Model file for the job. Use its own axes, mm. Face numbers are marked on the shaded views. A direction names the side the tool comes from. Round coordinates to 2 decimals unless told otherwise and drop trailing zeros. Loops run counter-clockwise (first coordinate to the right, second up) from the corner with the lowest first, then second, coordinate; pieces in that order, holes last. Notation, with made-up numbers: (-18.5, 30.25) - (17.5, 30.25) arc R24 ccw to (17.5, 64.25) - close; hole circle Ø4 at (29, 53.5). An arc over 180 degrees is marked (long way). Use one line per item in the form item = value.
from build123d import *

# Parameters (mm, degrees)
SKETCH1_W                      = 38.1
SKETCH1_H                      = 48.26
SKETCH1_W_2                    = 31.75
SKETCH1_H_2                    = 41.91
BOSS_EXTRUDE1_DEPTH            = 152.4
SKETCH2_R                      = 1.89865
CUT_EXTRUDE1_DEPTH             = 35.925
CUT_EXTRUDE1_DEPTH_BACK        = 4.175
CUT_EXTRUDE3_DEPTH             = 3.175
CUT_EXTRUDE4_DEPTH             = 3.175
CUT_EXTRUDE5_REACH             = 36.925
SKETCH6_R                      = 9.525
SKETCH6_R_2                    = 2.5527
CUT_EXTRUDE6_DEPTH             = 3.175
F_6_32_TAPPED_HOLE2_D          = 2.7051
F_6_32_TAPPED_HOLE2_DEPTH      = 3.175
CUT_EXTRUDE7_REACH             = 40.1
CUT_EXTRUDE7_DIRECTION_2_DEPTH = 1
FILLET1_R                      = 3.175
FILLET2_R                      = 3.175
BOSS_EXTRUDE2_DEPTH            = 3.175
CUT_EXTRUDE8_REACH             = 40.1
FILLET3_R                      = 3.175
FILLET4_R                      = 3.175
FILLET5_R                      = 6.35
FILLET6_R                      = 6.35
BOSS_EXTRUDE3_DEPTH            = 3.175
CUT_EXTRUDE9_REACH             = 40.1
BOSS_EXTRUDE4_DEPTH            = 3.175
FILLET7_R                      = 3.175
FILLET8_R                      = 3.175
FILLET9_R                      = 3.175
FILLET10_R                     = 3.175
FILLET11_R                     = 6.35
FILLET12_R                     = 6.35


with BuildPart() as part:
    # Sketch1 → Boss-Extrude1 (new body)
    with BuildSketch(Plane(origin=(0, 0, 0), x_dir=(1, 0, 0), z_dir=(0, 1, 0))):
        Rectangle(SKETCH1_W, SKETCH1_H)
        Rectangle(SKETCH1_W_2, SKETCH1_H_2, mode=Mode.SUBTRACT)
    extrude(amount=BOSS_EXTRUDE1_DEPTH)

    # Sketch2 → Cut-Extrude1 (cut, two sides)
    with BuildSketch(Plane(origin=(-15.875, 0, 0), x_dir=(0, 0, -1), z_dir=(1, 0, 0))) as cut_extrude1_sk:
        with Locations((-16.645384182, 6.21538)):
            Circle(SKETCH2_R)
        with Locations((10.30030417, 6.18241423)):
            Circle(SKETCH2_R)
    extrude(amount=CUT_EXTRUDE1_DEPTH, mode=Mode.SUBTRACT)
    extrude(cut_extrude1_sk.sketch, amount=-CUT_EXTRUDE1_DEPTH_BACK, mode=Mode.SUBTRACT)

    # Sketch4 → Cut-Extrude3 (cut)
    with BuildSketch(Plane.ZY.offset(19.05)):
        with BuildLine():
            Line((16.1925, 10.16), (-16.1925, 10.16))
            ThreePointArc((-16.1925, 10.16), (-18.43756403, 11.08993597), (-19.3675, 13.335))
            Line((-19.3675, 13.335), (-19.3675, 64.135))
            ThreePointArc((-19.3675, 64.135), (-18.43756403, 66.38006403), (-16.1925, 67.31))
            Line((-16.1925, 67.31), (16.1925, 67.31))
            ThreePointArc((16.1925, 67.31), (18.43756403, 66.38006403), (19.3675, 64.135))
            Line((19.3675, 64.135), (19.3675, 13.335))
            ThreePointArc((19.3675, 13.335), (18.43756403, 11.08993597), (16.1925, 10.16))
        make_face()
    extrude(amount=-CUT_EXTRUDE3_DEPTH, mode=Mode.SUBTRACT)

    # Sketch5 → Cut-Extrude4 (cut)
    with BuildSketch(Plane(origin=(19.05, 0, 0), x_dir=(0, 0, -1), z_dir=(1, 0, 0))):
        with BuildLine():
            Line((16.1925, 67.31), (-16.1925, 67.31))
            ThreePointArc((-16.1925, 67.31), (-18.43756403, 66.38006403), (-19.3675, 64.135))
            Line((-19.3675, 64.135), (-19.3675, 45.085))
            ThreePointArc((-19.3675, 45.085), (-18.43756403, 42.83993597), (-16.1925, 41.91))
            Line((-16.1925, 41.91), (16.1925, 41.91))
            ThreePointArc((16.1925, 41.91), (18.43756403, 42.83993597), (19.3675, 45.085))
            Line((19.3675, 45.085), (19.3675, 64.135))
            ThreePointArc((19.3675, 64.135), (18.43756403, 66.38006403), (16.1925, 67.31))
        make_face()
    extrude(amount=-CUT_EXTRUDE4_DEPTH, mode=Mode.SUBTRACT)

    # Sketch6 → Cut-Extrude5 (cut, up to next)
    with BuildSketch(Plane(origin=(-15.875, 0, 0), x_dir=(0, 0, -1), z_dir=(1, 0, 0)), mode=Mode.PRIVATE) as cut_extrude5_sk1:
        with Locations((0, 101.6)):
            Circle(SKETCH6_R)
    cut_extrude5_tool1 = extrude(cut_extrude5_sk1.sketch, amount=CUT_EXTRUDE5_REACH, mode=Mode.PRIVATE) & part.part
    add(cut_extrude5_tool1.solids().sort_by_distance((-15.875, 101.6, 0))[0], mode=Mode.SUBTRACT)
    # Sketch6 → Cut-Extrude5 (cut, up to next)
    with BuildSketch(Plane(origin=(-15.875, 0, 0), x_dir=(0, 0, -1), z_dir=(1, 0, 0)), mode=Mode.PRIVATE) as cut_extrude5_sk2:
        with Locations((0, 87.63)):
            Circle(SKETCH6_R_2)
    cut_extrude5_tool2 = extrude(cut_extrude5_sk2.sketch, amount=CUT_EXTRUDE5_REACH, mode=Mode.PRIVATE) & part.part
    add(cut_extrude5_tool2.solids().sort_by_distance((-15.875, 87.63, 0))[0], mode=Mode.SUBTRACT)
    # Sketch6 → Cut-Extrude5 (cut, up to next)
    with BuildSketch(Plane(origin=(-15.875, 0, 0), x_dir=(0, 0, -1), z_dir=(1, 0, 0)), mode=Mode.PRIVATE) as cut_extrude5_sk3:
        with Locations((-9.878281733, 91.721718267)):
            Circle(SKETCH6_R_2)
    cut_extrude5_tool3 = extrude(cut_extrude5_sk3.sketch, amount=CUT_EXTRUDE5_REACH, mode=Mode.PRIVATE) & part.part
    add(cut_extrude5_tool3.solids().sort_by_distance((-15.875, 91.721718, 9.878282))[0], mode=Mode.SUBTRACT)
    # Sketch6 → Cut-Extrude5 (cut, up to next)
    with BuildSketch(Plane(origin=(-15.875, 0, 0), x_dir=(0, 0, -1), z_dir=(1, 0, 0)), mode=Mode.PRIVATE) as cut_extrude5_sk4:
        with Locations((-13.97, 101.6)):
            Circle(SKETCH6_R_2)
    cut_extrude5_tool4 = extrude(cut_extrude5_sk4.sketch, amount=CUT_EXTRUDE5_REACH, mode=Mode.PRIVATE) & part.part
    add(cut_extrude5_tool4.solids().sort_by_distance((-15.875, 101.6, 13.97))[0], mode=Mode.SUBTRACT)
    # Sketch6 → Cut-Extrude5 (cut, up to next)
    with BuildSketch(Plane(origin=(-15.875, 0, 0), x_dir=(0, 0, -1), z_dir=(1, 0, 0)), mode=Mode.PRIVATE) as cut_extrude5_sk5:
        with Locations((-9.878281733, 111.478281733)):
            Circle(SKETCH6_R_2)
    cut_extrude5_tool5 = extrude(cut_extrude5_sk5.sketch, amount=CUT_EXTRUDE5_REACH, mode=Mode.PRIVATE) & part.part
    add(cut_extrude5_tool5.solids().sort_by_distance((-15.875, 111.478282, 9.878282))[0], mode=Mode.SUBTRACT)
    # Sketch6 → Cut-Extrude5 (cut, up to next)
    with BuildSketch(Plane(origin=(-15.875, 0, 0), x_dir=(0, 0, -1), z_dir=(1, 0, 0)), mode=Mode.PRIVATE) as cut_extrude5_sk6:
        with Locations((0, 115.57)):
            Circle(SKETCH6_R_2)
    cut_extrude5_tool6 = extrude(cut_extrude5_sk6.sketch, amount=CUT_EXTRUDE5_REACH, mode=Mode.PRIVATE) & part.part
    add(cut_extrude5_tool6.solids().sort_by_distance((-15.875, 115.57, 0))[0], mode=Mode.SUBTRACT)
    # Sketch6 → Cut-Extrude5 (cut, up to next)
    with BuildSketch(Plane(origin=(-15.875, 0, 0), x_dir=(0, 0, -1), z_dir=(1, 0, 0)), mode=Mode.PRIVATE) as cut_extrude5_sk7:
        with Locations((9.878281733, 111.478281733)):
            Circle(SKETCH6_R_2)
    cut_extrude5_tool7 = extrude(cut_extrude5_sk7.sketch, amount=CUT_EXTRUDE5_REACH, mode=Mode.PRIVATE) & part.part
    add(cut_extrude5_tool7.solids().sort_by_distance((-15.875, 111.478282, -9.878282))[0], mode=Mode.SUBTRACT)
    # Sketch6 → Cut-Extrude5 (cut, up to next)
    with BuildSketch(Plane(origin=(-15.875, 0, 0), x_dir=(0, 0, -1), z_dir=(1, 0, 0)), mode=Mode.PRIVATE) as cut_extrude5_sk8:
        with Locations((13.97, 101.6)):
            Circle(SKETCH6_R_2)
    cut_extrude5_tool8 = extrude(cut_extrude5_sk8.sketch, amount=CUT_EXTRUDE5_REACH, mode=Mode.PRIVATE) & part.part
    add(cut_extrude5_tool8.solids().sort_by_distance((-15.875, 101.6, -13.97))[0], mode=Mode.SUBTRACT)
    # Sketch6 → Cut-Extrude5 (cut, up to next)
    with BuildSketch(Plane(origin=(-15.875, 0, 0), x_dir=(0, 0, -1), z_dir=(1, 0, 0)), mode=Mode.PRIVATE) as cut_extrude5_sk9:
        with Locations((9.878281733, 91.721718267)):
            Circle(SKETCH6_R_2)
    cut_extrude5_tool9 = extrude(cut_extrude5_sk9.sketch, amount=CUT_EXTRUDE5_REACH, mode=Mode.PRIVATE) & part.part
    add(cut_extrude5_tool9.solids().sort_by_distance((-15.875, 91.721718, -9.878282))[0], mode=Mode.SUBTRACT)

    # Sketch7 → Cut-Extrude6 (cut)
    with BuildSketch(Plane.ZY.offset(19.05)):
        with BuildLine():
            Line((-13.0175, 77.47), (13.0175, 77.47))
            ThreePointArc((13.0175, 77.47), (17.507628061, 79.329871939), (19.3675, 83.82))
            Line((19.3675, 83.82), (19.3675, 121.92))
            ThreePointArc((19.3675, 121.92), (17.507628061, 126.410128061), (13.0175, 128.27))
            Line((13.0175, 128.27), (-13.0175, 128.27))
            ThreePointArc((-13.0175, 128.27), (-17.507628061, 126.410128061), (-19.3675, 121.92))
            Line((-19.3675, 121.92), (-19.3675, 83.82))
            ThreePointArc((-19.3675, 83.82), (-17.507628061, 79.329871939), (-13.0175, 77.47))
        make_face()
    extrude(amount=-CUT_EXTRUDE6_DEPTH, mode=Mode.SUBTRACT)

    # #6-32 Tapped Hole2
    with Locations(Plane(origin=(5.579615818, 136.6393, -24.13), x_dir=(-1, 0, 0), z_dir=(0, 0, -1))):
        with Locations((0, 0), (11.159231636, 0)):
            Hole(F_6_32_TAPPED_HOLE2_D / 2, depth=F_6_32_TAPPED_HOLE2_DEPTH)

    # Sketch13 → Cut-Extrude7 (cut, up to next)
    with BuildSketch(Plane(origin=(19.05, 0, 0), x_dir=(0, 0, -1), z_dir=(1, 0, 0)), mode=Mode.PRIVATE) as cut_extrude7_sk1:
        Polygon((0, 78.486), (19.3675, 78.486), (19.3675, 64.135), (-19.3675, 64.135), (-19.3675, 78.486), align=None)
    cut_extrude7_tool1 = extrude(cut_extrude7_sk1.sketch, amount=-CUT_EXTRUDE7_REACH, mode=Mode.PRIVATE) & part.part
    add(cut_extrude7_tool1.solids().sort_by_distance((19.05, 71.3105, 0))[0], mode=Mode.SUBTRACT)

    # Sketch13 → Cut-Extrude7 direction 2 (cut)
    with BuildSketch(Plane(origin=(19.05, 0, 0), x_dir=(0, 0, -1), z_dir=(1, 0, 0))):
        Polygon((0, 78.486), (19.3675, 78.486), (19.3675, 64.135), (-19.3675, 64.135), (-19.3675, 78.486), align=None)
    extrude(amount=CUT_EXTRUDE7_DIRECTION_2_DEPTH, mode=Mode.SUBTRACT)

    # Fillet1
    fillet1_edges = [part.edges().sort_by_distance(p)[0] for p in [
        (17.4625, 78.486, -19.3675),
    ]]
    fillet(fillet1_edges, radius=FILLET1_R)

    # Fillet2
    fillet2_edges = [part.edges().sort_by_distance(p)[0] for p in [
        (17.4625, 78.486, 19.3675),
    ]]
    fillet(fillet2_edges, radius=FILLET2_R)

    # Sketch15 → Boss-Extrude2 (add)
    with BuildSketch(Plane.ZY.offset(19.05)):
        Polygon((0, 78.486), (-19.3675, 78.486), (-19.3675, 88.646), (0, 88.646), (19.3675, 88.646), (19.3675, 78.486), align=None)
    extrude(amount=-BOSS_EXTRUDE2_DEPTH)

    # Sketch16 → Cut-Extrude8 (cut, up to next)
    with BuildSketch(Plane.ZY.offset(19.05), mode=Mode.PRIVATE) as cut_extrude8_sk1:
        Polygon((0, 78.486), (19.3675, 78.486), (19.3675, 64.135), (-19.3675, 64.135), (-19.3675, 78.486), align=None)
    cut_extrude8_tool1 = extrude(cut_extrude8_sk1.sketch, amount=-CUT_EXTRUDE8_REACH, mode=Mode.PRIVATE) & part.part
    add(cut_extrude8_tool1.solids().sort_by_distance((-19.05, 71.3105, 0))[0], mode=Mode.SUBTRACT)

    # Fillet3
    fillet3_edges = [part.edges().sort_by_distance(p)[0] for p in [
        (-17.4625, 78.486, 19.3675),
    ]]
    fillet(fillet3_edges, radius=FILLET3_R)

    # Fillet4
    fillet4_edges = [part.edges().sort_by_distance(p)[0] for p in [
        (-17.4625, 78.486, -19.3675),
    ]]
    fillet(fillet4_edges, radius=FILLET4_R)

    # Fillet5
    fillet5_edges = [part.edges().sort_by_distance(p)[0] for p in [
        (-17.4625, 88.646, -19.3675),
    ]]
    fillet(fillet5_edges, radius=FILLET5_R)

    # Fillet6
    fillet6_edges = [part.edges().sort_by_distance(p)[0] for p in [
        (-17.4625, 88.646, 19.3675),
    ]]
    fillet(fillet6_edges, radius=FILLET6_R)

    # Sketch17 → Boss-Extrude3 (add)
    with BuildSketch(Plane.ZY.offset(19.05)):
        Polygon((0, 74.168), (19.3675, 74.168), (19.3675, 84.35471455), (-20.6375, 84.35471455), (-19.3675, 74.168), align=None)
    extrude(amount=-BOSS_EXTRUDE3_DEPTH)

    # Sketch18 → Cut-Extrude9 (cut, up to next)
    with BuildSketch(Plane.ZY.offset(19.05), mode=Mode.PRIVATE) as cut_extrude9_sk1:
        Polygon((0, 84.328), (-19.3675, 84.328), (-19.3675, 94.996), (19.3675, 94.996), (19.3675, 84.328), align=None)
    cut_extrude9_tool1 = extrude(cut_extrude9_sk1.sketch, amount=-CUT_EXTRUDE9_REACH, mode=Mode.PRIVATE) & part.part
    add(cut_extrude9_tool1.solids().sort_by_distance((-19.05, 89.662, 0))[0], mode=Mode.SUBTRACT)

    # Sketch19 → Boss-Extrude4 (add)
    with BuildSketch(Plane(origin=(19.05, 0, 0), x_dir=(0, 0, -1), z_dir=(1, 0, 0))):
        Polygon((0, 74.168), (19.3675, 74.168), (19.3675, 78.486), (-19.3675, 78.486), (-19.3675, 74.168), align=None)
    extrude(amount=-BOSS_EXTRUDE4_DEPTH)

    # Fillet7
    fillet7_edges = [part.edges().sort_by_distance(p)[0] for p in [
        (17.4625, 74.168, -19.3675),
    ]]
    fillet(fillet7_edges, radius=FILLET7_R)

    # Fillet8
    fillet8_edges = [part.edges().sort_by_distance(p)[0] for p in [
        (17.4625, 74.168, 19.3675),
    ]]
    fillet(fillet8_edges, radius=FILLET8_R)

    # Fillet9
    fillet9_edges = [part.edges().sort_by_distance(p)[0] for p in [
        (-17.4625, 74.168, 19.3675),
    ]]
    fillet(fillet9_edges, radius=FILLET9_R)

    # Fillet10
    fillet10_edges = [part.edges().sort_by_distance(p)[0] for p in [
        (-17.4625, 74.168, -19.3675),
    ]]
    fillet(fillet10_edges, radius=FILLET10_R)

    # Fillet11
    fillet11_edges = [part.edges().sort_by_distance(p)[0] for p in [
        (-17.4625, 84.328, -19.3675),
    ]]
    fillet(fillet11_edges, radius=FILLET11_R)

    # Fillet12
    fillet12_edges = [part.edges().sort_by_distance(p)[0] for p in [
        (-17.4625, 84.328, 19.3675),
    ]]
    fillet(fillet12_edges, radius=FILLET12_R)


solid = part.part
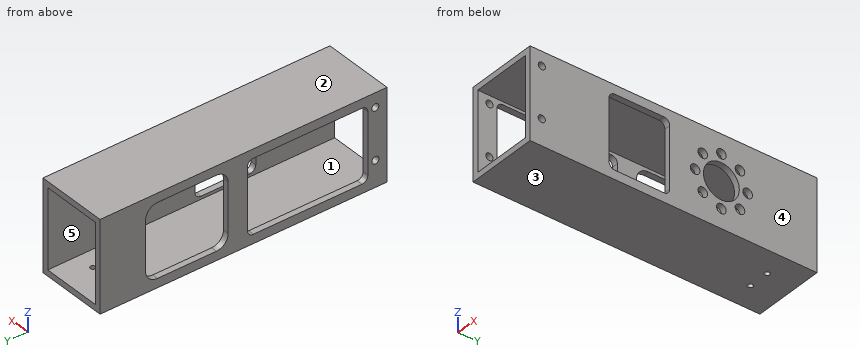
1. Flat gauge pins, fed straight in: pin 1 (3 mm diameter, centred on x = -5.58, y = 136.64, fed in from -Z); pin 2 (2 mm diameter, centred on y = 28.5, z = -8.5, fed in from -X) (3 decimals). Where does each tip first touch, or does it go through?
Geometry check:
pin_1 = -24.13
pin_2 = 15.875
2. Tool access for the marked faces 4 and 5: list every direction of +Z, -Z, +X, -X, +Y, -Y with a clear straight run to the whole face (end or side of a thin tool).
Geometry check:
face_4 = +Z, -Z, +X, +Y, -Y
face_5 = +Y, -Y
3. Cut at B-B, the plane z = 0. Give the number of separate pieces and of enclosed holes in the cut face, plus the area to 3 significant figures.
Geometry check:
separate_pieces = 8
enclosed_holes = 0
area = 430 mm^2
4. Cut at D-D, the plane y = 78. Give the cut face in (x, z) (3 decimals), plus the area to 3 significant figures.
Geometry check:
outline = (-19.05, -24.13) - (19.05, -24.13) - (19.05, 24.13) - (-19.05, 24.13) - close; hole (-15.875, -20.955) - (15.875, -20.955) - (15.875, 20.955) - (-15.875, 20.955) - close
area = 508 mm^2
5. Cut at A-A, the plane x = 1.5. Give the cut face in (y, z) (3 decimals), plus the area to 3 significant figures.
Geometry check:
outline = (0, -24.13) - (152.4, -24.13) - (152.4, -20.955) - (0, -20.955) - close; (0, 20.955) - (152.4, 20.955) - (152.4, 24.13) - (0, 24.13) - close
area = 968 mm^2
6. Wall check: probe 1 along Y at (x, z) = (16.85, 0) (3 decimals); probe 2 along Z at (x, y) = (16.7, 101.6) (3 decimals); probe 3 along X at (y, z) = (6.5, 2) (3 decimals). Give the ranges that are in metal, low to high.
Geometry check:
probe_1 = 0 to 41.91, 74.168 to 85.077, 90.183 to 92.075, 111.125 to 113.017, 118.123 to 152.4
probe_2 = -24.13 to -16.523, -11.417 to -9.525, 9.525 to 11.417, 16.523 to 24.13
probe_3 = -19.05 to -15.875, 15.875 to 19.05
7. Pull direction Z, two halves, no side cores. Call the marked faces 1, 2 and 3: +Z half, -Z half, draft (parallel to the pull), parting line (faces both ways), or undercut.
Geometry check:
face_1 = undercut
face_2 = +Z half
face_3 = -Z half
